```python
from build123d import *

# Parameters (mm, degrees)
BOSS_EXTRU_1_DEPTH      = 10
BOSS_EXTRU_3_DEPTH      = 13
ENL_V_MAT_EXTRU_1_DEPTH = 31.702233225
BOSS_EXTRU_4_DEPTH      = 2
CHANFREIN1_SIZE         = 2
CHANFREIN2_SIZE         = 0.5


with BuildPart() as part:
    # Esquisse1 → Boss.-Extru.1 (new body)
    with BuildSketch(Plane(origin=(0, 0, 0), x_dir=(0, 1, 0), z_dir=(0, 0, 1))):
        with BuildLine():
            Line((-7.89, -10.855), (-7.89, 10.855))
            ThreePointArc((-7.89, 10.855), (0, 18.745), (7.89, 10.855))
            Line((7.89, 10.855), (7.89, -10.855))
            ThreePointArc((7.89, -10.855), (0, -18.745), (-7.89, -10.855))
        make_face()
    extrude(amount=BOSS_EXTRU_1_DEPTH)

    # Esquisse3 → Boss.-Extru.3 (add)
    with BuildSketch(Plane(origin=(0, 0, 0), x_dir=(1, 0, 0), z_dir=(0, 0, -1))):
        Polygon((10.855, -3.695041723), (14.055, -1.847520861), (14.055, 1.847520861), (10.855, 3.695041723), (7.655, 1.847520861), (7.655, -1.847520861), align=None)
    extrude(amount=BOSS_EXTRU_3_DEPTH)

    # Esquisse2 → Enlèv. mat.-Extru.1 (cut, through all)
    with BuildSketch(Plane.XY.offset(10)):
        Polygon((-10.855, 3.935), (-14.262809964, 1.9675), (-14.262809964, -1.9675), (-10.855, -3.935), (-7.447190036, -1.9675), (-7.447190036, 1.9675), align=None)
    extrude(amount=-ENL_V_MAT_EXTRU_1_DEPTH, mode=Mode.SUBTRACT)

    # Esquisse4 → Boss.-Extru.4 (add)
    with BuildSketch(Plane.XY.offset(10)):
        with BuildLine():
            ThreePointArc((-10.855, -7.89), (-5.275927496, -5.579072504), (-2.965, 0))
            ThreePointArc((-2.965, 0), (-5.275927496, 5.579072504), (-10.855, 7.89))
            ThreePointArc((-10.855, 7.89), (-18.745, 0), (-10.855, -7.89))
        make_face()
        Polygon((-10.855, 3.935), (-7.447190036, 1.9675), (-7.447190036, -1.9675), (-10.855, -3.935), (-14.262809964, -1.9675), (-14.262809964, 1.9675), align=None, mode=Mode.SUBTRACT)
    extrude(amount=BOSS_EXTRU_4_DEPTH)

    # Chanfrein1
    chanfrein1_edges = [part.edges().sort_by_distance(p)[0] for p in [
        (-9.151095018, 2.95125, 12),
        (-7.447190036, 0, 12),
        (-9.151095018, -2.95125, 12),
        (-12.558904982, -2.95125, 12),
        (-14.262809964, 0, 12),
        (-12.558904982, 2.95125, 12),
    ]]
    chamfer(chanfrein1_edges, length=CHANFREIN1_SIZE - 0.0001)  # a hair under: the kernel refuses the full size

    # Chanfrein2
    chanfrein2_edges = [part.edges().sort_by_distance(p)[0] for p in [
        (9.255, 2.771281292, -13),
        (12.455, 2.771281292, -13),
        (14.055, 0, -13),
        (12.455, -2.771281292, -13),
        (9.255, -2.771281292, -13),
        (7.655, 0, -13),
    ]]
    chamfer(chanfrein2_edges, length=CHANFREIN2_SIZE)


solid = part.part
```
Input: part model. Units: mm. Frame: model coordinates. A direction names the side the tool comes from. Coordinates: 2 decimals unless noted, no trailing zeros. Loops run counter-clockwise (first coordinate to the right, second up) from the corner with the lowest first, then second, coordinate; pieces in that order, holes last. Notation, with made-up numbers: M -39,2.5 L 10,2.5 A24 ccw 10,25.5 Z; hole C 6.25,84 d4. An arc over 180 degrees is marked long. Answer in a Markdown table with one row per item.
1. Section B-B, the plane z = -6. Output: boundary loops of the cut face in (x, y) (3 decimals), then the cut area to 3 significant figures.
Response:
| item | result |
|---|---|
| outline | M 7.655,-1.848 L 10.855,-3.695 L 14.055,-1.848 L 14.055,1.848 L 10.855,3.695 L 7.655,1.848 Z |
| area | 35.5 mm2 |
2. Section D-D, the plane x = 10. Output: boundary loops of the cut face in (y, z), then the cut area to 3 significant figures.
Response:
| item | result |
|---|---|
| outline | M -7.89,0 L -3.2,0 L -3.2,-12.5 L -2.62,-13 L 2.62,-13 L 3.2,-12.5 L 3.2,0 L 7.89,0 L 7.89,10 L -7.89,10 Z |
| area | 241 mm2 |
3. Reachability of faces 4 (the flat face through (-15.25, -0.04, 10.99)), 5 (the flat face through (14.055, 0, -6)), 6 (the flat face through (-12.535, -2.965, 4.93)) from +Z, -Z, +X, -X, +Y, -Y: full face, straight path, thin tool, end or side. Return the list, or none.
Response:
| item | result |
|---|---|
| face 4 | +Z |
| face 5 | -Z, +X, +Y, -Y |
| face 6 | +Z, -Z |
4. Draft query along X for faces 1 (the flat face through (-13.014, -3.827, 10.986)), 2 (the flat face through (9.233, 2.758, -6.162)), 3 (the flat face through (12.477, -2.758, -6.162)). Return one class per face: pulls with the +X half, pulls with the -X half, needs draft (parallel to the pull), parting line crosses it, or undercut.
Response:
| item | result |
|---|---|
| face 1 | undercut |
| face 2 | pulls with the -X half |
| face 3 | pulls with the +X half |
5. Material intervals for line 1 (Z direction, x = -0.5, y = 2.5); line 2 (Z direction, x = -5.5, y = -4.5); line 3 (X direction, y = 0, z = 7.25) (3 decimals), sorted ascending.
Response:
| item | result |
|---|---|
| line 1 | z = 0 to 10 |
| line 2 | z = 0 to 12 |
| line 3 | x = -18.745 to -14.263, -7.447 to 18.745 |
6. Section C-C, the plane y = -2.5. Output: boundary loops of the cut face in (x, z), then the cut area to 3 significant figures.
Response:
| item | result |
|---|---|
| outline | M -18.34,0 L -13.34,0 L -13.34,10 L -15.19,10.92 L -16.26,12 L -18.34,12 Z; M -8.37,0 L 8.79,0 L 8.79,-12.5 L 9.79,-13 L 11.92,-13 L 12.92,-12.5 L 12.92,0 L 18.34,0 L 18.34,10 L -3.37,10 L -3.37,12 L -5.45,12 L -6.52,10.92 L -8.37,10 Z |
| area | 384 mm2 |
7. Section A-A, the plane z = 0.5. Output: boundary loops of the cut face in (x, y) (1 decimal), then the cut area to 3 significant figures.
Response:
| item | result |
|---|---|
| outline | M -10.9,-7.9 L 10.9,-7.9 A7.9 ccw 10.9,7.9 L -10.9,7.9 A7.9 ccw Z; hole M -14.3,-2 L -10.9,-3.9 L -7.4,-2 L -7.4,2 L -10.9,3.9 L -14.3,2 Z |
| area | 498 mm2 |
8. First-contact query: pin 1 (1.5 mm diameter, centred on x = -12, y = -0.5, fed in from -Z); pin 2 (8 mm diameter, centred on x = -6, y = 1.5, fed in from -Z); pin 3 (1.8 mm diameter, centred on y = -0.5, z = -4, fed in from +X) (3 decimals); pin 4 (3 mm diameter, centred on x = 13, z = 5, fed in from -Y). Flat tips, straight axial feed; report the tip coordinate or a pass-through.
Response:
| item | result |
|---|---|
| pin 1 | passes through |
| pin 2 | stops at z = 0 |
| pin 3 | stops at x = 14.055 |
| pin 4 | stops at y = -7.86 |
